```python
from build123d import *

# Parameters (mm, degrees)
F0_R     = 53.9496
F1_DEPTH = 6.35
F2_R     = 25.9715
F3_DEPTH = 3.175
F4_R     = 17.4625
F5_DEPTH = 9.526
F6_D     = 7.1374


with BuildPart() as f1:
    # F0 (on Right) → F1 (new body)
    with BuildSketch(Plane.YZ):
        Circle(F0_R)
    extrude(amount=-F1_DEPTH)

    # F2 (on face) → F3 (join)
    with BuildSketch(Plane(origin=(-6.35, 0, 0), x_dir=(0, -1, 0), z_dir=(-1, 0, 0))):
        Circle(F2_R)
    extrude(amount=F3_DEPTH)

    # F4 (on face) → F5 (cut, through all)
    with BuildSketch(Plane.YZ):
        Circle(F4_R)
    extrude(amount=-F5_DEPTH, mode=Mode.SUBTRACT)

    # F6 (through all)
    with Locations(Plane.YZ):
        with Locations((0, -44.45), (44.45, 0), (0, 44.45), (-44.45, 0)):
            Hole(F6_D / 2)


solid = f1.part
```
Here's how the part is built. I have some questions about the finished solid (model axes, mm). A direction names the side the tool comes from. Round coordinates to 2 decimals unless told otherwise and drop trailing zeros. Loops run counter-clockwise (first coordinate to the right, second up) from the corner with the lowest first, then second, coordinate; pieces in that order, holes last. Notation, with made-up numbers: (44.25, 58) -> (94.25, 58) arc R20 ccw to (94.25, 91) -> close; hole circle Ø6 at (64, -26). An arc over 180 degrees is marked (long way). Answer as CSV lines item,"result".
1. Thinking about a two-plate mould opening in Y: for faces 3 (the face through (-3.131, -11.695, -52.667)), 4 (the face through (-9.525, -17, -5)), 5 (the face through (-3.22, 0.46, -40.91)), which applies, released by +Y, released by -Y, zero draft, split by the parting line, or undercut?
Final values:
face 3,"split by the parting line"
face 4,"zero draft"
face 5,"undercut"
2. If we section it at A-A on y = 0: Count the separate pieces of the cut face and the enclosed holes in it, plus the area to 3 significant figures.
Final values:
separate pieces,"4"
enclosed holes,"0"
area,"427 mm^2"
3. Which directions (+Z, -Z, +X, -X, +Y, -Y) give clear straight access to the entire face, cutting with the end or side of a thin tool? Please do faces 1 (the face through (-3.219, 48.015, 0.157)), 2 (the face through (-6.35, 23, 13)).
Final values:
face 1,"+X, -X"
face 2,"-X"
4. For pin 1 (4.5 mm diameter, centred on y = -44.45, z = 0, fed in from -X); pin 2 (2 mm diameter, centred on y = -20.5, z = -33.5, fed in from -X); pin 3 (1 mm diameter, centred on x = -5.5, z = -42, fed in from -Y); pin 4 (1.5 mm diameter, centred on x = -6, y = -36, fed in from -Z), each with a flat end and sliding along its axis, tell me the tip position at first contact or that it passes through.
Final values:
pin 1,"passes through"
pin 2,"stops at x = -6.35"
pin 3,"stops at y = -34.47"
pin 4,"stops at z = -40.84"
5. If we section it at C-C on z = -44.45: Please give me the cut outline in (x, y), plus the area to 3 significant figures.
Final values:
outline,"(-6.35, -30.57) -> (0, -30.57) -> (0, -3.57) -> (-6.35, -3.57) -> close; (-6.35, 3.57) -> (0, 3.57) -> (0, 30.57) -> (-6.35, 30.57) -> close"
area,"343 mm^2"
6. If I drill on L1, parallel to Z at x = -6.75, y = 0; L2, parallel to Z at x = -2.25, y = 0; L3, parallel to X at y = 28, z = 32, over which ranges is the centre line in solid material (lowest first)?
Final values:
L1,"z = -25.97 to -17.46, 17.46 to 25.97"
L2,"z = -53.95 to -48.02, -40.88 to -17.46, 17.46 to 40.88, 48.02 to 53.95"
L3,"x = -6.35 to 0"
